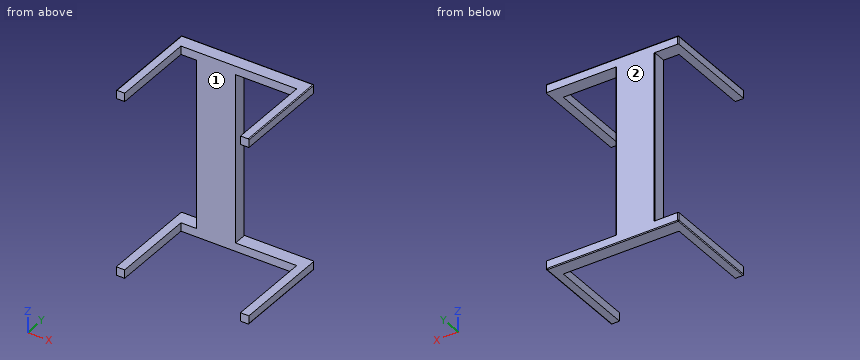
from build123d import *

# Parameters (mm, degrees)
CROQUIS1_W              = 1000
CROQUIS1_H              = 740
SALIENTE_EXTRUIR1_DEPTH = 1400
CROQUIS2_W              = 873
CROQUIS2_H              = 638.4
CORTAR_EXTRUIR1_DEPTH   = 1400
CROQUIS3_W              = 1273
CROQUIS3_H              = 638.4
CORTAR_EXTRUIR2_DEPTH   = 1000
CROQUIS4_W              = 180
CROQUIS4_H              = 1273
CROQUIS4_W_2            = 525
CORTAR_EXTRUIR3_DEPTH   = 200
REDONDEO1_R             = 6
REDONDEO2_R             = 6
REDONDEO4_R             = 6


with BuildPart() as part:
    # Croquis1 → Saliente-Extruir1 (new body)
    with BuildSketch(Plane.XY):
        with Locations((500, -370)):
            Rectangle(CROQUIS1_W, CROQUIS1_H)
    extrude(amount=SALIENTE_EXTRUIR1_DEPTH)

    # Croquis2 → Cortar-Extruir1 (cut)
    with BuildSketch(Plane.XY.offset(1400)):
        with Locations((500, -420.8)):
            Rectangle(CROQUIS2_W, CROQUIS2_H)
    extrude(amount=-CORTAR_EXTRUIR1_DEPTH, mode=Mode.SUBTRACT)

    # Croquis3 → Cortar-Extruir2 (cut)
    with BuildSketch(Plane(origin=(1000, 0, 0), x_dir=(0, 0, -1), z_dir=(1, 0, 0))):
        with Locations((-700, -420.8)):
            Rectangle(CROQUIS3_W, CROQUIS3_H)
    extrude(amount=-CORTAR_EXTRUIR2_DEPTH, mode=Mode.SUBTRACT)

    # Croquis4 → Cortar-Extruir3 (cut)
    with BuildSketch(Plane(origin=(0, 0, 0), x_dir=(1, 0, 0), z_dir=(0, 1, 0))):
        with Locations((90, -700)):
            Rectangle(CROQUIS4_W, CROQUIS4_H)
        with Locations((737.5, -700)):
            Rectangle(CROQUIS4_W_2, CROQUIS4_H)
    extrude(amount=-CORTAR_EXTRUIR3_DEPTH, mode=Mode.SUBTRACT)

    # Redondeo1
    redondeo1_edges = [part.edges().sort_by_distance(p)[0] for p in [
        (0, 0, 31.75),
        (0, 0, 1368.25),
        (1000, 0, 1368.25),
        (1000, 0, 31.75),
    ]]
    fillet(redondeo1_edges, radius=REDONDEO1_R)

    # Redondeo2
    redondeo2_edges = [part.edges().sort_by_distance(p)[0] for p in [
        (180, 0, 700),
        (475, 0, 700),
    ]]
    fillet(redondeo2_edges, radius=REDONDEO2_R)

    # Redondeo4
    redondeo4_edges = [part.edges().sort_by_distance(p)[0] for p in [
        (1000, -373, 1400),
        (0, -373, 1400),
        (500, 0, 0),
        (500, 0, 1400),
        (998.242640687, -1.757359313, 1400),
        (1.757359313, -1.757359313, 1400),
        (0, -373, 0),
        (998.242640687, -1.757359313, 0),
        (1.757359313, -1.757359313, 0),
        (1000, -373, 0),
    ]]
    fillet(redondeo4_edges, radius=REDONDEO4_R)


solid = part.part
Check sheet for the modelled part. Datum: model origin and axes. Units: mm. Face numbers are marked on the shaded views. Round coordinates to 2 decimals unless told otherwise and drop trailing zeros. Order: outer loops, then holes, each group sorted by start corner. A loop starts at its lowest first (then second) coordinate and runs counter-clockwise, first axis right, second up.
Q1. Draft check along X on the marked faces 1 and 2. Enter one of: pulls with the +X half, pulls with the -X half, needs draft (parallel to the pull), parting line crosses it, or undercut.
Filled sheet:
face 1: undercut
face 2: needs draft
Q2. Depth check by flat-ended pin: P1, Ø10, axis at x = 237.5, z = 562, coming from the -Y side. Enter the tip coordinate at first touch or a pass-through.
Filled sheet:
P1: stops at y = -101.6
Q3. Cross-section at C-C, the plane y = -58. Enter the section's corners in (x, z), plus the area to 3 significant figures.
Filled sheet:
outline: (0, 6) arc R6 ccw to (6, 0) - (994, 0) arc R6 ccw to (1000, 6) - (1000, 63.5) - (475, 63.5) - (475, 1336.5) - (1000, 1336.5) - (1000, 1394) arc R6 ccw to (994, 1400) - (6, 1400) arc R6 ccw to (0, 1394) - (0, 1336.5) - (180, 1336.5) - (180, 63.5) - (0, 63.5) - close
area: 503,000 mm2
Q4. Cross-section at A-A, the plane y = -226. Enter the section's corners in (x, z).
Filled sheet:
outline: (0, 6) arc R6 ccw to (6, 0) - (63.5, 0) - (63.5, 63.5) - (0, 63.5) - close; (0, 1336.5) - (63.5, 1336.5) - (63.5, 1400) - (6, 1400) arc R6 ccw to (0, 1394) - close; (936.5, 0) - (994, 0) arc R6 ccw to (1000, 6) - (1000, 63.5) - (936.5, 63.5) - close; (936.5, 1336.5) - (1000, 1336.5) - (1000, 1394) arc R6 ccw to (994, 1400) - (936.5, 1400) - close
Q5. Scan lines: L1, parallel to Z at x = 552, y = -62.5; L2, parallel to Y at x = 349, z = 1192; L3, parallel to X at y = -59, z = 509. Record each from-to range of solid material in increasing order.
Filled sheet:
L1: z = 0 to 63.5, 1336.5 to 1400
L2: y = -101.6 to 0
L3: x = 180 to 475
Q6. Cross-section at B-B, the plane x = 498. Enter the section's corners in (y, z).
Filled sheet:
outline: (-101.6, 0) - (-6, 0) arc R6 ccw to (0, 6) - (0, 63.5) - (-101.6, 63.5) - close; (-101.6, 1336.5) - (0, 1336.5) - (0, 1394) arc R6 ccw to (-6, 1400) - (-101.6, 1400) - close
Q7. Cross-section at D-D, the plane z = 1152. Enter the section's corners in (x, y), plus the area to 3 significant figures.
Filled sheet:
outline: (180, -101.6) - (475, -101.6) - (475, -6) arc R6 ccw to (469, 0) - (186, 0) arc R6 ccw to (180, -6) - close
area: 30,000 mm2
